from build123d import *

# Parameters (mm, degrees)
F0_W      = 2000
F0_H      = 1000
F1_DEPTH  = 25
F2_W      = 100
F2_H      = 100
F3_DEPTH  = 700
F4_R      = 25
F5_DEPTH  = 100
F6_W      = 100
F6_H      = 100
F7_DEPTH  = 700
F8_R      = 25
F9_DEPTH  = 100
F10_W     = 100
F10_H     = 100
F11_DEPTH = 700
F12_R     = 25
F13_DEPTH = 100
F14_W     = 100
F14_H     = 100
F15_DEPTH = 700
F16_R     = 25
F17_DEPTH = 100
F19_DEPTH = 25


with BuildPart() as f1:
    # F0 (on Top) → F1 (new body)
    with BuildSketch(Plane.XY):
        with Locations((7.790016, -81.412016)):
            Rectangle(F0_W, F0_H)
    extrude(amount=F1_DEPTH)

    # F2 (on face) → F3 (join)
    with BuildSketch(Plane.XY.offset(25)):
        with Locations((-892.209984, 318.587984)):
            Rectangle(F2_W, F2_H)
    extrude(amount=F3_DEPTH)

    # F4 (on face) → F5 (cut)
    with BuildSketch(Plane(origin=(0, 368.587984, 0), x_dir=(-1, 0, 0), z_dir=(0, 1, 0))):
        with Locations((892.209984, 125)):
            Circle(F4_R)
        with Locations((892.209984, 325)):
            Circle(F4_R)
        with Locations((892.209984, 525)):
            Circle(F4_R)
    extrude(amount=-F5_DEPTH, mode=Mode.SUBTRACT)

    # F6 (on face) → F7 (join)
    with BuildSketch(Plane.XY.offset(25)):
        with Locations((907.790016, 318.587984)):
            Rectangle(F6_W, F6_H)
    extrude(amount=F7_DEPTH)

    # F8 (on face) → F9 (cut)
    with BuildSketch(Plane(origin=(0, 368.587984, 0), x_dir=(-1, 0, 0), z_dir=(0, 1, 0))):
        with Locations((-907.790016, 125)):
            Circle(F8_R)
        with Locations((-907.790016, 325)):
            Circle(F8_R)
        with Locations((-907.790016, 525)):
            Circle(F8_R)
    extrude(amount=-F9_DEPTH, mode=Mode.SUBTRACT)

    # F10 (on face) → F11 (join)
    with BuildSketch(Plane.XY.offset(25)):
        with Locations((-892.209984, -481.412016)):
            Rectangle(F10_W, F10_H)
    extrude(amount=F11_DEPTH)

    # F12 (on face) → F13 (cut)
    with BuildSketch(Plane.XZ.offset(531.412016)):
        with Locations((-892.209984, 525)):
            Circle(F12_R)
        with Locations((-892.209984, 325)):
            Circle(F12_R)
        with Locations((-892.209984, 125)):
            Circle(F12_R)
    extrude(amount=-F13_DEPTH, mode=Mode.SUBTRACT)

    # F14 (on face) → F15 (join)
    with BuildSketch(Plane.XY.offset(25)):
        with Locations((907.790016, -481.412016)):
            Rectangle(F14_W, F14_H)
    extrude(amount=F15_DEPTH)

    # F16 (on face) → F17 (cut)
    with BuildSketch(Plane.XZ.offset(531.412016)):
        with Locations((907.790016, 525)):
            Circle(F16_R)
        with Locations((907.790016, 325)):
            Circle(F16_R)
        with Locations((907.790016, 125)):
            Circle(F16_R)
    extrude(amount=-F17_DEPTH, mode=Mode.SUBTRACT)

    # F18 (on face) → F19 (cut)
    with BuildSketch(Plane(origin=(0, 0, 0), x_dir=(1, 0, 0), z_dir=(0, 0, -1))):
        with BuildLine():
            Line((-411.143931, -418.587984), (337.688116, -418.587984))
            ThreePointArc((337.688116, -418.587984), (-36.727907, -269.433703), (-411.143931, -418.587984))
        make_face()
    extrude(amount=-F19_DEPTH, mode=Mode.SUBTRACT)


solid = f1.part
Geometry check sheet. Reference: the model listing, model coordinates, mm. A direction names the side the tool comes from. Give positions to 0.01 mm unless a question says otherwise; leave off trailing zeros. Order: outer loops, then holes, each group sorted by start corner. A loop starts at its lowest first (then second) coordinate and runs counter-clockwise, first axis right, second up.
1. Scan lines: line 1 (Z direction, x = -337, y = -239); line 2 (X direction, y = 288.5, z = 430). Record each from-to range of solid material in increasing order.
Completed:
line 1: z = 0 to 25
line 2: x = -942.21 to -842.21, 857.79 to 957.79
2. Draft check along Z on faces 1 (the face through (-867.234, 319.288, 326.099)), 2 (the face through (-893, 319, 725)), 3 (the face through (-942.21, -482, 370)). Enter one of: pulls with the +Z half, pulls with the -Z half, needs draft (parallel to the pull), parting line crosses it, or undercut.
Completed:
face 1: undercut
face 2: pulls with the +Z half
face 3: needs draft
3. Sectioned sample at B-B (x = 435). Record the boundary of the cut face in (y, z).
Completed:
outline: (-581.41, 0) - (418.59, 0) - (418.59, 25) - (-581.41, 25) - close
4. Access from +Z, -Z, +X, -X, +Y, -Y to the whole of each face (thin tool, end or side, straight path). Record for faces 4 (the face through (957.79, -482, 370)), 5 (the face through (-868.364, -482.112, 532.509)), 6 (the face through (907, 368.588, 370)), 7 (the face through (-942.21, 318, 370)), 8 (the face through (-842.21, -482, 370)).
Completed:
face 4: +Z, +X, +Y, -Y
face 5: +Y, -Y
face 6: +Z, +X, -X, +Y
face 7: +Z, -X, +Y, -Y
face 8: +Z, +Y, -Y
5. Sectioned sample at A-A (z = 525). State how many separate pieces and enclosed holes the cut face has, then the cut area to 3 significant figures.
Completed:
separate pieces: 8
enclosed holes: 0
area: 20,000 mm2
6. Sectioned sample at C-C (y = 63.5). Record the boundary of the cut face in (x, z), then the cut area to 3 significant figures.
Completed:
outline: (-992.21, 0) - (1007.79, 0) - (1007.79, 25) - (-992.21, 25) - close
area: 50,000 mm2
